Check sheet for the modelled part. Datum: model origin and axes. Units: mm. Face numbers are marked on the shaded views. A direction names the side the tool comes from. Round coordinates to 2 decimals unless told otherwise and drop trailing zeros. Write each loop counter-clockwise with the first axis right and the second up, starting at its lowest first coordinate (ties: lowest second). Pieces come first, ordered by that corner, then holes. Notation, with made-up numbers: (87, -37) - (107, -37) arc R25 ccw to (107, -12) - close; hole circle Ø7 at (71, 19). An arc over 180 degrees is marked (long way). Use one line per item in the form item = value. Start each with the question number.
1) Section check B-B (x = 0). Record the boundary of the cut face in (y, z), then the cut area to 3 significant figures.
2) Section check D-D (x = 3). Record the boundary of the cut face in (y, z), then the cut area to 3 significant figures.
3) Gauge pin test, flat ends, axial feed: P1, Ø8, axis at x = 7.5, z = 9.5, coming from the -Y side; P2, Ø12.5, axis at x = -2, y = -20.5, coming from the -Z side; P3, Ø6, axis at x = -2.5, y = -5.5, coming from the -Z side. Record the tip position at first contact, or that the pin passes through.
4) Section check C-C (z = 13). Record the boundary of the cut face in (x, y).
5) Scan lines: probe 1 along Y at (x, z) = (0, 12.65); probe 2 along Y at (x, z) = (1, 12.25); probe 3 along Z at (x, y) = (-3.5, -42). Record each from-to range of solid material in increasing order.
6) Section check A-A (y = -35). Record the boundary of the cut face in (x, z), then the cut area to 3 significant figures.
7) Set-up check for the marked faces 1, 2 and 3: record each of +Z, -Z, +X, -X, +Y, -Y from which the full face is reachable in a straight line by a thin tool's end or side.
8) Draft check along Y on the marked faces 4, 5, 6 and 7. Enter one of: +Y half, -Y half, draft (parallel to the pull), parting line (faces both ways), or undercut.
from build123d import *

# Parameters (mm, degrees)
SKETCH_1_R      = 2.5
EXTRUDE_1_DEPTH = 11
EXTRUDE_2_DEPTH = 3
EXTRUDE_START   = -3
SKETCH_4_R      = 10
SKETCH_4_R_2    = 6.5
EXTRUDE_3_DEPTH = 3
FILLET_START    = 11
FILLET_1_DEPTH  = 3


with BuildPart() as part:
    # 草图1 → 凸台-拉伸1 (new body)
    with BuildSketch(Plane.XY):
        Circle(SKETCH_1_R)
    extrude(amount=EXTRUDE_1_DEPTH)

    # 草图2 → 旋转1 (revolve)
    with BuildSketch(Plane(origin=(0, 0, 0), x_dir=(1, 0, 0), z_dir=(0, 1, 0))):
        with BuildLine():
            Line((0, 0), (-4.358898944, 0))
            ThreePointArc((-4.358898944, 0), (-2.236067977, 0.746794345), (0, 1))
            Line((0, 1), (0, 0))
        make_face()
    revolve(axis=Axis((0, 0, 0), (0, 0, -1)))

    # 草图3 → 凸台-拉伸2 (add)
    with BuildSketch(Plane.XY.offset(11)):
        with BuildLine():
            Line((-4.883855118, 1.071428571), (-12.209637796, -32.321428571))
            ThreePointArc((-12.209637796, -32.321428571), (0, -47.5), (12.209637796, -32.321428571))
            Line((12.209637796, -32.321428571), (4.883855118, 1.071428571))
            ThreePointArc((4.883855118, 1.071428571), (0, 5), (-4.883855118, 1.071428571))
        make_face()
        with BuildLine():
            Line((-9.767710237, -32.857142857), (-4.883855118, -10.595238095))
            ThreePointArc((-4.883855118, -10.595238095), (0, -6.666666667), (4.883855118, -10.595238095))
            Line((4.883855118, -10.595238095), (9.767710237, -32.857142857))
            ThreePointArc((9.767710237, -32.857142857), (0, -45), (-9.767710237, -32.857142857))
        make_face(mode=Mode.SUBTRACT)
    extrude(amount=EXTRUDE_2_DEPTH)

    # 草图4 → 凸台-拉伸3 (add)
    with BuildSketch(Plane.XY.offset(14).offset(EXTRUDE_START)):
        with Locations((0, -35)):
            Circle(SKETCH_4_R)
        with Locations((0, -35)):
            Circle(SKETCH_4_R_2, mode=Mode.SUBTRACT)
    extrude(amount=EXTRUDE_3_DEPTH)

    # 圆角1: read off the stored shape, not the designer's step
    # 圆角1 outline → 圆角1 (add)
    with BuildSketch(Plane.XY.offset(FILLET_START)):
        with BuildLine():
            ThreePointArc((6.737252603, -19.043514567), (5.547910317, -23.48400457), (1.235598323, -25.076628759))
            ThreePointArc((1.235598323, -25.076628759), (6.738122863, -27.610974335), (9.767710237, -32.857142857))
            Line((9.767710237, -32.857142857), (6.737252603, -19.043514567))
        make_face()
        with BuildLine():
            ThreePointArc((-9.767710237, -32.857142857), (-6.738122863, -27.610974335), (-1.235598323, -25.076628759))
            ThreePointArc((-1.235598323, -25.076628759), (-5.547910317, -23.48400457), (-6.737252603, -19.043514567))
            Line((-6.737252603, -19.043514567), (-9.767710237, -32.857142857))
        make_face()
    extrude(amount=FILLET_1_DEPTH)


solid = part.part
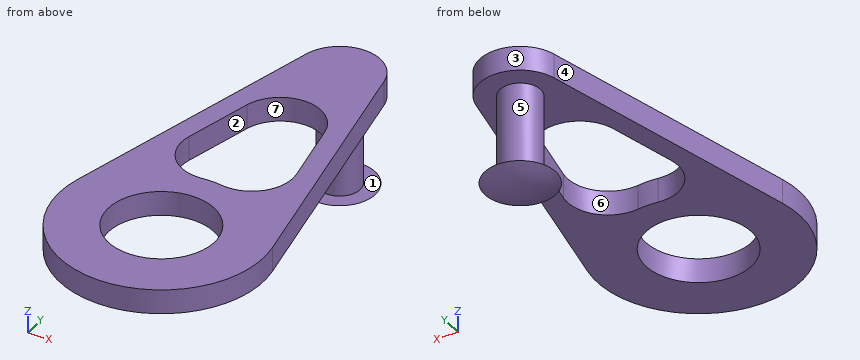
Results are:
q1.outline = (-47.5, 11) - (-41.5, 11) - (-41.5, 14) - (-47.5, 14) - close; (-28.5, 11) - (-25, 11) - (-25, 14) - (-28.5, 14) - close; (-6.67, 11) - (-2.5, 11) - (-2.5, 0) - (-4.36, 0) arc R10 ccw to (4.36, 0) - (2.5, 0) - (2.5, 11) - (5, 11) - (5, 14) - (-6.67, 14) - close
q1.area = 124 mm²
q2.outline = (-47.13, 11) - (-40.77, 11) - (-40.77, 14) - (-47.13, 14) - close; (-29.23, 11) - (-24.98, 11) - (-24.98, 14) - (-29.23, 14) - close; (-7.67, 11) - (4, 11) - (4, 14) - (-7.67, 14) - close; (-3.16, 0) arc R9.54 ccw to (3.16, 0) - close
q2.area = 69.1 mm²
q3.P1 = -46.91
q3.P2 = 11
q3.P3 = -0.53
q4.outline = (-12.21, -32.32) arc R12.5 ccw (long way) to (12.21, -32.32) - (4.88, 1.07) arc R5 ccw to (-4.88, 1.07) - close; hole (-6.74, -19.04) arc R5 ccw to (-1.24, -25.08) arc R10 cw to (1.24, -25.08) arc R5 ccw to (6.74, -19.04) - (4.88, -10.6) arc R5 ccw to (-4.88, -10.6) - close; hole circle Ø13 at (0, -35)
q5.probe_1 = -47.5 to -41.5, -28.5 to -25, -6.67 to 5
q5.probe_2 = -47.46 to -41.42, -28.58 to -25.05, -6.77 to 4.9
q5.probe_3 = 11 to 14
q6.outline = (-12.5, 11) - (-6.5, 11) - (-6.5, 14) - (-12.5, 14) - close; (6.5, 11) - (12.5, 11) - (12.5, 14) - (6.5, 14) - close
q6.area = 36.0 mm²
q7.face_1 = none
q7.face_2 = +Z, -Z
q7.face_3 = +Z, -Z, +Y
q8.face_4 = +Y half
q8.face_5 = parting line
q8.face_6 = undercut
q8.face_7 = undercut
